```python
from build123d import *

# Parameters (mm, degrees)
MODEL_R                 = 8.05
MODEL_R_2               = 1
MODEL_W                 = 5
MODEL_H                 = 5
MODEL_W_2               = 11.8
MODEL_H_2               = 22.5
SALIENTE_EXTRUIR1_DEPTH = 3
CROQUIS2_R              = 1.5
CORTAR_EXTRUIR1_DEPTH   = 1
CROQUIS4_W              = 19.999967436
CROQUIS4_H              = 3
SALIENTE_EXTRUIR2_DEPTH = 8
CROQUIS5_R              = 1.5
CORTAR_EXTRUIR2_DEPTH   = 3
REDONDEO1_R             = 2
CROQUIS6_R              = 12
CORTAR_EXTRUIR3_DEPTH   = 1


with BuildPart() as part:
    # Model → Saliente-Extruir1 (new body)
    with BuildSketch(Plane.XY):
        with BuildLine():
            Line((28.600020379, -36.098945331), (29.600020379, -36.098945331))
            ThreePointArc((29.600020379, -36.098945331), (30.307127161, -35.806052112), (30.600020379, -35.098945331))
            Line((30.600020379, -35.098945331), (30.600020379, 4.974420659))
            ThreePointArc((30.600020379, 4.974420659), (33.150320304, 10.94136051), (38.69115159, 14.318872844))
            ThreePointArc((38.69115159, 14.318872844), (38.049426695, 11.673196605), (38.544127303, 8.99613013))
            ThreePointArc((38.544127303, 8.99613013), (43.872924224, 13.634815248), (50.51172433, 16.051385009))
            ThreePointArc((50.51172433, 16.051385009), (49.487728366, 13.546636971), (50.534778199, 11.051438157))
            ThreePointArc((50.534778199, 11.051438157), (55.112285588, 14.426569266), (60.460332405, 16.361376528))
            ThreePointArc((60.460332405, 16.361376528), (62.537747107, 11.66270114), (66.497154818, 8.389126209))
            ThreePointArc((66.497154818, 8.389126209), (73.089038309, 12.831206377), (80.665288642, 15.236499516))
            ThreePointArc((80.665288642, 15.236499516), (82.62970299, 7.967186508), (89.013428278, 3.973455574))
            ThreePointArc((89.013428278, 3.973455574), (90.223089011, 3.212884764), (90.943701038, 1.979002536))
            Line((90.943701038, 1.979002536), (90.943701038, -35.070997464))
            ThreePointArc((90.943701038, -35.070997464), (91.236594257, -35.778104245), (91.943701038, -36.070997464))
            Line((91.943701038, -36.070997464), (92.943701038, -36.070997464))
            ThreePointArc((92.943701038, -36.070997464), (93.650807819, -35.778104245), (93.943701038, -35.070997464))
            Line((93.943701038, -35.070997464), (93.943701038, -21.120997464))
            ThreePointArc((93.943701038, -21.120997464), (94.529487475, -19.706783901), (95.943701038, -19.120997464))
            Line((95.943701038, -19.120997464), (109.743701038, -19.120997464))
            ThreePointArc((109.743701038, -19.120997464), (111.1579146, -19.706783901), (111.743701038, -21.120997464))
            Line((111.743701038, -21.120997464), (111.743701038, -51.020997464))
            ThreePointArc((111.743701038, -51.020997464), (111.1579146, -52.435211026), (109.743701038, -53.020997464))
            Line((109.743701038, -53.020997464), (72.771860709, -53.020997464))
            ThreePointArc((72.771860709, -53.020997464), (71.357647146, -53.606783901), (70.771860709, -55.020997464))
            Line((70.771860709, -55.020997464), (70.771860709, -56.020573856))
            Line((70.771860709, -56.020573856), (50.771893273, -56.020573856))
            Line((50.771893273, -56.020573856), (50.771882418, -55.020552149))
            ThreePointArc((50.771882418, -55.020552149), (50.186088306, -53.606352619), (48.771882419, -53.020573857))
            Line((48.771882419, -53.020573857), (11.743679941, -53.020573857))
            ThreePointArc((11.743679941, -53.020573857), (10.369303805, -52.451275514), (9.800020379, -51.076893199))
            Line((9.800020379, -51.076893199), (9.800020379, -21.120997464))
            ThreePointArc((9.800020379, -21.120997464), (10.385806817, -19.706783901), (11.800020379, -19.120997464))
            Line((11.800020379, -19.120997464), (25.600020379, -19.120997464))
            ThreePointArc((25.600020379, -19.120997464), (27.014233942, -19.706783901), (27.600020379, -21.120997464))
            Line((27.600020379, -21.120997464), (27.600020379, -35.098945331))
            ThreePointArc((27.600020379, -35.098945331), (27.892913598, -35.806052112), (28.600020379, -36.098945331))
        make_face()
        with Locations((47.698959583, -8.020997464)):
            Circle(MODEL_R, mode=Mode.SUBTRACT)
        with Locations((73.698959582, -8.020997464)):
            Circle(MODEL_R, mode=Mode.SUBTRACT)
        with Locations((102.770799912, -49.020997464)):
            Circle(MODEL_R_2, mode=Mode.SUBTRACT)
        with Locations((102.770799912, -21.720997464)):
            Circle(MODEL_R_2, mode=Mode.SUBTRACT)
        with Locations((18.627119253, -49.020997464)):
            Circle(MODEL_R_2, mode=Mode.SUBTRACT)
        with Locations((18.627119253, -21.720997464)):
            Circle(MODEL_R_2, mode=Mode.SUBTRACT)
        Polygon((53.283896073, -43.364264203), (57.614023092, -45.864264203), (60.114023092, -41.534137185), (55.783896073, -39.034137185), align=None, mode=Mode.SUBTRACT)
        Polygon((63.783896073, -45.864264204), (68.114023092, -43.364264204), (65.614023092, -39.034137185), (61.283896073, -41.534137185), align=None, mode=Mode.SUBTRACT)
        with Locations((68.698959582, -35.520997464)):
            Rectangle(MODEL_W, MODEL_H, mode=Mode.SUBTRACT)
        Polygon((68.114023092, -27.677730724), (63.783896073, -25.177730724), (61.283896073, -29.507857743), (65.614023092, -32.007857743), align=None, mode=Mode.SUBTRACT)
        Polygon((57.614023092, -25.177730724), (53.283896073, -27.677730724), (55.783896073, -32.007857743), (60.114023092, -29.507857743), align=None, mode=Mode.SUBTRACT)
        with Locations((52.698959582, -35.520997464)):
            Rectangle(MODEL_W, MODEL_H, mode=Mode.SUBTRACT)
        Polygon((58.198975864, -33.020997464), (58.344778117, -38.020997464), (63.198975864, -38.020997464), (63.198975864, -33.020997464), align=None, mode=Mode.SUBTRACT)
        with Locations((102.770799912, -35.370997464)):
            Rectangle(MODEL_W_2, MODEL_H_2, mode=Mode.SUBTRACT)
        with Locations((18.627119253, -35.370997464)):
            Rectangle(MODEL_W_2, MODEL_H_2, mode=Mode.SUBTRACT)
    extrude(amount=SALIENTE_EXTRUIR1_DEPTH)

    # Croquis2 → Cortar-Extruir1 (cut)
    with BuildSketch(Plane.XY.offset(3)):
        with Locations((18.627119253, -21.720997464)):
            Circle(CROQUIS2_R)
        with Locations((18.627119253, -49.020997464)):
            Circle(CROQUIS2_R)
        with Locations((102.770799912, -49.020997464)):
            Circle(CROQUIS2_R)
        with Locations((102.770799912, -21.720997464)):
            Circle(CROQUIS2_R)
    extrude(amount=-CORTAR_EXTRUIR1_DEPTH, mode=Mode.SUBTRACT)

    # Croquis4 → Saliente-Extruir2 (add)
    with BuildSketch(Plane(origin=(0, 0, 0), x_dir=(-1, 0, 0), z_dir=(0, 0, -1))):
        with Locations((-60.771876991, -54.520573856)):
            Rectangle(CROQUIS4_W, CROQUIS4_H)
    extrude(amount=SALIENTE_EXTRUIR2_DEPTH)

    # Croquis5 → Cortar-Extruir2 (cut)
    with BuildSketch(Plane(origin=(0, -53.020573856, 0), x_dir=(1, 0, 0), z_dir=(0, 1, 0))):
        with Locations((66.771876991, 3.5)):
            Circle(CROQUIS5_R)
        with Locations((54.771876991, 3.5)):
            Circle(CROQUIS5_R)
    extrude(amount=-CORTAR_EXTRUIR2_DEPTH, mode=Mode.SUBTRACT)

    # Redondeo1
    redondeo1_edges = [part.edges().sort_by_distance(p)[0] for p in [
        (50.771893273, -54.520573856, -8),
        (70.771860709, -54.520573856, -8),
    ]]
    fillet(redondeo1_edges, radius=REDONDEO1_R)

    # Croquis6 → Cortar-Extruir3 (cut)
    with BuildSketch(Plane(origin=(0, 0, 0), x_dir=(-1, 0, 0), z_dir=(0, 0, -1))):
        with Locations((-60.771860709, -35.520573857)):
            Circle(CROQUIS6_R)
    extrude(amount=-CORTAR_EXTRUIR3_DEPTH, mode=Mode.SUBTRACT)


solid = part.part
```
Input: part model. Units: mm. Frame: model coordinates. A direction names the side the tool comes from. Round coordinates to 2 decimals unless told otherwise and drop trailing zeros. Order: outer loops, then holes, each group sorted by start corner. A loop starts at its lowest first (then second) coordinate and runs counter-clockwise, first axis right, second up. Notation, with made-up numbers: (62, -12.75) - (104, -12.75) arc R30 ccw to (104, 20.25) - close; hole circle Ø11 at (32.25, 1). An arc over 180 degrees is marked (long way). Answer in a Markdown table with one row per item.
Item 1: Line query: line 1 (X direction, y = -54.95, z = -3.5); line 2 (X direction, y = 11.5, z = 1.5); line 3 (X direction, y = -40.5, z = 2). Output: solid intervals per line, ascending.
Model answer:
| item | result |
|---|---|
| line 1 | x = 50.77 to 53.27, 56.27 to 65.27, 68.27 to 70.77 |
| line 2 | x = 33.67 to 38.05, 40.93 to 50.15, 51 to 62.66, 70.65 to 80.94 |
| line 3 | x = 9.8 to 12.73, 24.53 to 54.94, 58.32 to 63.08, 66.46 to 96.87, 108.67 to 111.74 |
Item 2: Pin query (flat end, axial travel): pin 1 (4 mm diameter, centred on x = 101.5, z = 1.5, fed in from -Y); pin 2 (2 mm diameter, centred on x = 53, z = 2.5, fed in from +Y); pin 3 (2.5 mm diameter, centred on x = 103.5, z = 2, fed in from +Y). Return the tip coordinate at first contact, or that it passes through.
Model answer:
| item | result |
|---|---|
| pin 1 | stops at y = -53.02 |
| pin 2 | stops at y = 13.78 |
| pin 3 | stops at y = -19.12 |
Item 3: Section query A-A (z = -3.5). Return the cut outline in (x, y).
Model answer:
| item | result |
|---|---|
| outline | (50.77, -56.02) - (53.27, -56.02) - (53.27, -53.02) - (50.77, -53.02) - close; (56.27, -56.02) - (65.27, -56.02) - (65.27, -53.02) - (56.27, -53.02) - close; (68.27, -56.02) - (70.77, -56.02) - (70.77, -53.02) - (68.27, -53.02) - close |
Item 4: Section query B-B (y = -14). Return the cut outline in (x, z), then the cut area to 3 significant figures.
Model answer:
| item | result |
|---|---|
| outline | (30.6, 0) - (42.31, 0) - (42.31, 3) - (30.6, 3) - close; (53.09, 0) - (68.31, 0) - (68.31, 3) - (53.09, 3) - close; (79.09, 0) - (90.94, 0) - (90.94, 3) - (79.09, 3) - close |
| area | 116 mm² |
Item 5: Reachability of faces 1 (the flat face through (54.55, -41.17, 1.99)), 2 (the cylindrical face through (27, -19.69, 1.48)), 3 (the flat face through (61, -53.021, -4)), 4 (the flat face through (61, -56.021, -2)), 5 (the flat face through (18, -50, 2)) from +Z, -Z, +X, -X, +Y, -Y: full face, straight path, thin tool, end or side. Return the list, or none.
Model answer:
| item | result |
|---|---|
| face 1 | +Z, -Z |
| face 2 | +Z, -Z, +Y |
| face 3 | -Z, +X, -X, +Y |
| face 4 | +Z, -Z, +X, -X, -Y |
| face 5 | +Z |
Item 6: Mould query, pull axis X, two halves, no side actions, for faces 6 (the flat face through (96.871, -36, 1)), 7 (the flat face through (19, -19.121, 1)), 8 (the cylindrical face through (90.209, 3.227, 1.479)), 9 (the cylindrical face through (10.37, -19.72, 1.48)). Classes: released by +X, released by -X, zero draft, split by the parting line, or undercut.
Model answer:
| item | result |
|---|---|
| face 6 | undercut |
| face 7 | zero draft |
| face 8 | released by +X |
| face 9 | released by -X |
